from build123d import *

# Parameters (mm, degrees)
SKETCH_1_R          = 40
EXTRUDE_1_DEPTH     = 4
SKETCH_2_R          = 5
SKETCH_2_R_2        = 1.5
CUT_EXTRUDE_1_DEPTH = 5


with BuildPart() as part:
    # 草图1 → 凸台-拉伸1 (new body)
    with BuildSketch(Plane.XY):
        Circle(SKETCH_1_R)
    extrude(amount=EXTRUDE_1_DEPTH)

    # 草图2 → 切除-拉伸1 (cut, through all)
    with BuildSketch(Plane.XY.offset(4)):
        Circle(SKETCH_2_R)
        with Locations((-8, 0)):
            Circle(SKETCH_2_R_2)
        with Locations((0, 8)):
            Circle(SKETCH_2_R_2)
        with Locations((8, 0)):
            Circle(SKETCH_2_R_2)
        with Locations((0, -8)):
            Circle(SKETCH_2_R_2)
        with BuildLine():
            Line((-3, 29.849623113), (-3, 12.649110641))
            ThreePointArc((-3, 12.649110641), (-11.258330249, 6.5), (-12.45445115, -3.726479109))
            Line((-12.45445115, -3.726479109), (-27.350531909, -12.326735345))
            ThreePointArc((-27.350531909, -12.326735345), (-25.980762114, 15), (-3, 29.849623113))
        make_face()
        with BuildLine():
            Line((3, 29.849623113), (3, 12.649110641))
            ThreePointArc((3, 12.649110641), (11.258330249, 6.5), (12.45445115, -3.726479109))
            Line((12.45445115, -3.726479109), (27.350531909, -12.326735345))
            ThreePointArc((27.350531909, -12.326735345), (25.980762114, 15), (3, 29.849623113))
        make_face()
        with BuildLine():
            Line((24.350531909, -17.522887768), (9.45445115, -8.922631532))
            ThreePointArc((9.45445115, -8.922631532), (0, -13), (-9.45445115, -8.922631532))
            Line((-9.45445115, -8.922631532), (-24.350531909, -17.522887768))
            ThreePointArc((-24.350531909, -17.522887768), (0, -30), (24.350531909, -17.522887768))
        make_face()
    extrude(amount=-CUT_EXTRUDE_1_DEPTH, mode=Mode.SUBTRACT)


solid = part.part
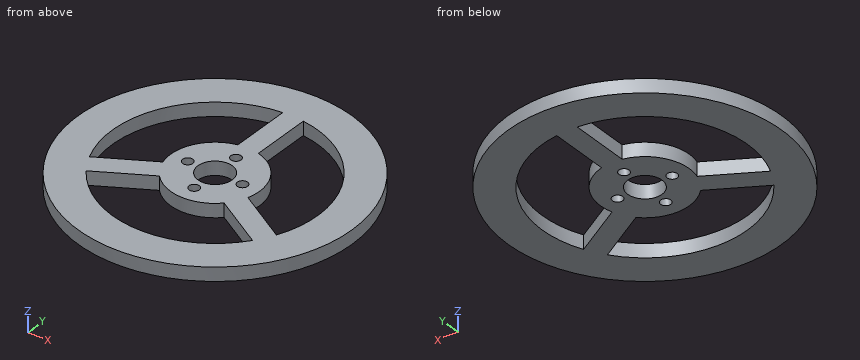
The model under review builds one solid part; all positions refer to its coordinate system, in mm. Coordinates: 2 decimals unless noted, no trailing zeros. Write each loop counter-clockwise with the first axis right and the second up, starting at its lowest first coordinate (ties: lowest second). Pieces come first, ordered by that corner, then holes. Notation, with made-up numbers: (3.25, -24) - (37.25, -24) arc R28 ccw to (37.25, 13) - close; hole circle Ø6 at (-22.5, 57.25). An arc over 180 degrees is marked (long way). Answer as a JSON object with one key per item and string values. Group by question number.
1. Add section B-B (y = 28). Give the boundary of the cut face in (x, z), plus the area to 3 significant figures.
2. To check wall thickness, follow probe 1 along Y at (x, z) = (0, 2.45); probe 2 along X at (y, z) = (7, 0.2); probe 3 along X at (y, z) = (18.5, 0.85). State the ranges of each line that lie inside material, in increasing order.
3. Add section D-D (z = 3.1). Give the number of separate pieces and of enclosed holes in the cut face, plus the area to 3 significant figures.
4. Add section A-A (x = 0). Give the boundary of the cut face in (y, z), plus the area to 3 significant figures.
5. Clearance check with flat-ended pins moving along their axes: pin 1 Ø2 at (y, z) = (21, 3) entering from -X; pin 2 Ø8 at (x, y) = (0, 0) entering from -Z; pin 3 Ø2 at (y, z) = (-4.5, 3) entering from +X; pin 4 Ø2 at (x, z) = (29, 1.5) entering from +Y. State where each tip first meets the part, or that it passes through.
6. Add section C-C (x = -8). Give the boundary of the cut face in (y, z), plus the area to 3 significant figures.
Findings:
{
 "1": {"outline": "(-28.57, 0) - (-10.77, 0) - (-10.77, 4) - (-28.57, 4) - close; (-3, 0) - (3, 0) - (3, 4) - (-3, 4) - close; (10.77, 0) - (28.57, 0) - (28.57, 4) - (10.77, 4) - close", "area": "166 mm²"},
 "2": {"probe 1": "-40 to -30, -13 to -9.5, -6.5 to -5, 5 to 6.5, 9.5 to 40", "probe 2": "-39.38 to -29.17, -10.95 to -1.12, 1.12 to 10.95, 29.17 to 39.38", "probe 3": "-35.46 to -23.62, -3 to 3, 23.62 to 35.46"},
 "3": {"separate pieces": "1", "enclosed holes": "8", "area": "2,930 mm²"},
 "4": {"outline": "(-40, 0) - (-30, 0) - (-30, 4) - (-40, 4) - close; (-13, 0) - (-9.5, 0) - (-9.5, 4) - (-13, 4) - close; (-6.5, 0) - (-5, 0) - (-5, 4) - (-6.5, 4) - close; (5, 0) - (6.5, 0) - (6.5, 4) - (5, 4) - close; (9.5, 0) - (40, 0) - (40, 4) - (9.5, 4) - close", "area": "188 mm²"},
 "5": {"pin 1": "x = -34.64", "pin 2": "through", "pin 3": "x = 39.85", "pin 4": "y = 28.57"},
 "6": {"outline": "(-39.19, 0) - (-28.91, 0) - (-28.91, 4) - (-39.19, 4) - close; (-10.25, 0) - (-1.5, 0) - (-1.5, 4) - (-10.25, 4) - close; (1.5, 0) - (10.25, 0) - (10.25, 4) - (1.5, 4) - close; (28.91, 0) - (39.19, 0) - (39.19, 4) - (28.91, 4) - close", "area": "152 mm²"}
}
